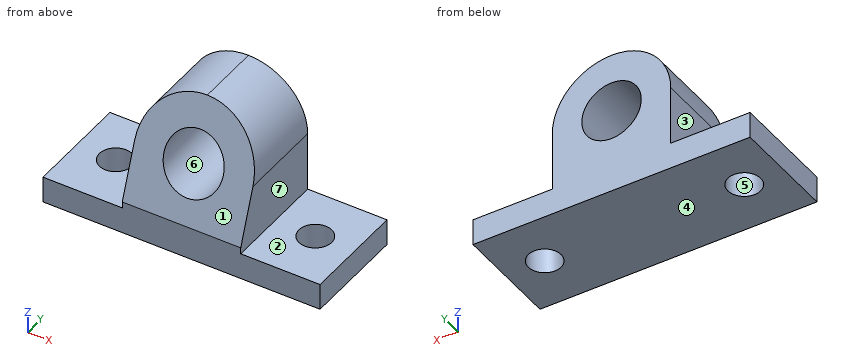
```python
from build123d import *

# Parameters (mm, degrees)
F0_W     = 50.8
F0_H     = 15.748
F1_DEPTH = 133.096
F2_R     = 14.2875
F3_DEPTH = 50.8
F4_R     = 7.874
F5_DEPTH = 12.7


with BuildPart() as f1:
    # F0 (on Right) → F1 (new body)
    with BuildSketch(Plane.YZ):
        Polygon((24.598954, 14.818944), (-6.601977, 14.818944), (-26.201046, -39.029056), (24.598954, -39.029056), align=None)
        with Locations((-0.801046, -46.903056)):
            Rectangle(F0_W, F0_H)
    extrude(amount=F1_DEPTH)

    # F2 (on face) → F3 (cut)
    with BuildSketch(Plane(origin=(0, 24.598954, 0), x_dir=(-1, 0, 0), z_dir=(0, 1, 0))):
        with BuildLine():
            Line((-133.096, 14.818944), (-133.096, -42.077056))
            Line((-133.096, -42.077056), (-94.996, -42.077056))
            Line((-94.996, -42.077056), (-94.996, -13.629056))
            ThreePointArc((-94.996, -13.629056), (-86.663774, 6.486718), (-66.548, 14.818944))
            Line((-66.548, 14.818944), (-133.096, 14.818944))
        make_face()
        with BuildLine():
            Line((-38.1, -42.077056), (0, -42.077056))
            Line((0, -42.077056), (0, 14.818944))
            Line((0, 14.818944), (-66.548, 14.818944))
            ThreePointArc((-66.548, 14.818944), (-46.432226, 6.486718), (-38.1, -13.629056))
            Line((-38.1, -13.629056), (-38.1, -42.077056))
        make_face()
        with Locations((-66.548, -13.629056)):
            Circle(F2_R)
    extrude(amount=-F3_DEPTH, mode=Mode.SUBTRACT)

    # F4 (on face) → F5 (cut)
    with BuildSketch(Plane(origin=(0, 0, -54.777056), x_dir=(1, 0, 0), z_dir=(0, 0, -1))):
        with Locations((18.796865, 0.687916)):
            Circle(F4_R)
        with Locations((114.299135, 0.11313)):
            Circle(F4_R)
    extrude(amount=-F5_DEPTH, mode=Mode.SUBTRACT)


solid = f1.part
```
Geometry: final body of the model. Coordinates: model frame, mm. Face numbers are marked on the shaded views. A direction names the side the tool comes from. Round coordinates to 2 decimals unless told otherwise and drop trailing zeros. Order: outer loops, then holes, each group sorted by start corner. A loop starts at its lowest first (then second) coordinate and runs counter-clockwise, first axis right, second up. Notation, with made-up numbers: M -13.5,29 L -2.5,29 A22 ccw -2.5,51 Z; hole C 66.25,-28 d11. An arc over 180 degrees is marked long. One line per item, written item: value.
(1) Cut plane C-C (z = -6.5). Return the cut outline in (x, y).
Result sheet:
outline: M 39.01,-14.36 L 54.17,-14.36 L 54.17,24.6 L 39.01,24.6 Z; M 78.93,-14.36 L 94.09,-14.36 L 94.09,24.6 L 78.93,24.6 Z
(2) Cut plane D-D (y = -2). Return the cut outline in (x, z) (1 decimal), and give its area (3 significant figures).
Result sheet:
outline: M 0,-54.8 L 11,-54.8 L 11,-42.1 L 0,-42.1 Z; M 26.6,-54.8 L 106.7,-54.8 L 106.7,-42.1 L 95,-42.1 L 95,-13.6 A28.4 ccw 66.5,14.8 A28.4 ccw 38.1,-13.6 L 38.1,-42.1 L 26.6,-42.1 Z; M 121.9,-54.8 L 133.1,-54.8 L 133.1,-42.1 L 121.9,-42.1 Z; hole C 66.5,-13.6 d28.6
area: 3,550 mm2
(3) Reachability of the marked faces 1, 2 and 3 from +Z, -Z, +X, -X, +Y, -Y: full face, straight path, thin tool, end or side. Return the list, or none.
Result sheet:
face 1: +Z, +X, -X, -Y
face 2: +Z, +X, +Y, -Y
face 3: +Z, -X, +Y, -Y
(4) Line query: probe 1 along X at (y, z) = (13, -13); probe 2 along Z at (x, y) = (33, -21); probe 3 along Y at (x, z) = (84.5, -39). Output: solid intervals per line, ascending. Write a range as [from, to].
Result sheet:
probe 1: [38.11, 52.27], [80.82, 94.99]
probe 2: [-54.78, -42.08]
probe 3: [-26.19, 24.6]
(5) Pin query (flat end, axial travel): P1, Ø2, axis at x = 48.5, z = -33, coming from the -Y side; P2, Ø25, axis at x = 18.8, y = -0.69, coming from the +Z side; P3, Ø23, axis at y = -9, z = -25.5, coming from the -X side. Return the tip coordinate at first contact, or that it passes through.
Result sheet:
P1: y = -24.37
P2: z = -42.08
P3: x = 38.1
(6) Cut plane A-A (y = 16.5). Return the cut outline in (x, z) (1 decimal), and give its area (3 significant figures).
Result sheet:
outline: M 0,-54.8 L 133.1,-54.8 L 133.1,-42.1 L 95,-42.1 L 95,-13.6 A28.4 ccw 66.5,14.8 A28.4 ccw 38.1,-13.6 L 38.1,-42.1 L 0,-42.1 Z; hole C 66.5,-13.6 d28.6
area: 3,940 mm2
(7) Pull-direction query (X, two-part tool) for the marked faces 4, 5, 6 and 7; classes: pulls with the +X half, pulls with the -X half, needs draft (parallel to the pull), parting line crosses it, or undercut.
Result sheet:
face 4: needs draft
face 5: undercut
face 6: undercut
face 7: pulls with the +X half
(8) Cut plane B-B (x = 119). Return the cut outline in (y, z).
Result sheet:
outline: M -26.2,-54.78 L -6.43,-54.78 L -6.43,-42.08 L -26.2,-42.08 Z; M 6.2,-54.78 L 24.6,-54.78 L 24.6,-42.08 L 6.2,-42.08 Z
